from build123d import *

# Parameters (mm, degrees)
F1_DEPTH = 8
F2_R     = 2.5
F2_R_2   = 2
F3_DEPTH = 25
F5_DEPTH = 4
F7_DEPTH = 3
F8_R     = 0.5
F9_R     = 0.5


# Not quite as in the source:
# - a feature names something its author has since deleted; it is built from what else it names


with BuildPart() as f1:
    # F0 (on Top) → F1 (new body)
    with BuildSketch(Plane.XY):
        with BuildLine():
            Line((6.4761662253, 49.1160303571), (6.5, 49.6721517667))
            ThreePointArc((6.5, 49.6721517667), (0, 56.1721517667), (-6.5, 49.6721517667))
            Line((-6.5, 49.6721517667), (-6.4761662253, 49.1160303571))
            ThreePointArc((-6.4761662253, 49.1160303571), (0, 43.1721517667), (6.4761662253, 49.1160303571))
        make_face()
        with BuildLine():
            ThreePointArc((6.4761662253, 49.1160303571), (6.4940388228, 49.3938358172), (6.5, 49.6721517667))
            Line((6.5, 49.6721517667), (6.4761662253, 49.1160303571))
        make_face()
        with BuildLine():
            Line((-6.4761662253, 49.1160303571), (-6.5, 49.6721517667))
            ThreePointArc((-6.5, 49.6721517667), (-6.4940388228, 49.3938358172), (-6.4761662253, 49.1160303571))
        make_face()
        with BuildLine():
            Line((5, 14.6721517667), (6.4761662253, 49.1160303571))
            ThreePointArc((6.4761662253, 49.1160303571), (0, 43.1721517667), (-6.4761662253, 49.1160303571))
            Line((-6.4761662253, 49.1160303571), (-5, 14.6721517667))
            ThreePointArc((-5, 14.6721517667), (0, 19.6721517667), (5, 14.6721517667))
        make_face()
        with BuildLine():
            ThreePointArc((-5, 14.6721517667), (0, 9.6721517667), (5, 14.6721517667))
            ThreePointArc((5, 14.6721517667), (0, 19.6721517667), (-5, 14.6721517667))
        make_face()
    extrude(amount=F1_DEPTH)

    # F2 (on face) → F3 (cut)
    with BuildSketch(Plane.XY.offset(8)):
        with Locations((0, 49.6721517667)):
            Circle(F2_R)
        with Locations((0, 14.6721517667)):
            Circle(F2_R_2)
    extrude(amount=-F3_DEPTH, mode=Mode.SUBTRACT)

    # F4 (on face) → F5 (cut)
    with BuildSketch(Plane.XY.offset(8)):
        with BuildLine():
            Line((3.84, 48.5521517667), (4, 49.6721517667))
            ThreePointArc((4, 49.6721517667), (0, 53.6721517667), (-4, 49.6721517667))
            Line((-4, 49.6721517667), (-3.8313540205, 48.522923169))
            ThreePointArc((-3.8313540205, 48.522923169), (0.0152402747, 45.6721808001), (3.84, 48.5521517667))
        make_face()
        with BuildLine():
            ThreePointArc((3.84, 48.5521517667), (3.9597979746, 49.1064663418), (4, 49.6721517667))
            Line((4, 49.6721517667), (3.84, 48.5521517667))
        make_face()
        with BuildLine():
            Line((-3.8313540205, 48.522923169), (-4, 49.6721517667))
            ThreePointArc((-4, 49.6721517667), (-3.9576139328, 49.0913833455), (-3.8313540205, 48.522923169))
        make_face()
        with BuildLine():
            Line((2, 35.6721517667), (3.84, 48.5521517667))
            ThreePointArc((3.84, 48.5521517667), (0.0152402747, 45.6721808001), (-3.8313540205, 48.522923169))
            Line((-3.8313540205, 48.522923169), (-1.9833417846, 35.929747119))
            ThreePointArc((-1.9833417846, 35.929747119), (0.1290667091, 37.6679828679), (2, 35.6721517667))
        make_face()
        with BuildLine():
            ThreePointArc((-1.9833417846, 35.929747119), (-0.1290667091, 33.6763206655), (2, 35.6721517667))
            ThreePointArc((2, 35.6721517667), (0.1290667091, 37.6679828679), (-1.9833417846, 35.929747119))
        make_face()
    extrude(amount=-F5_DEPTH, mode=Mode.SUBTRACT)

    # F6 (on face) → F7 (cut)
    with BuildSketch(Plane.XY.offset(8)):
        with BuildLine():
            ThreePointArc((-4.1204651564, 17.5044241573), (0, 19.6721517667), (4.1204651564, 17.5044241573))
            Line((4.1204651564, 17.5044241573), (4.8918937278, 35.5044241573))
            ThreePointArc((4.8918937278, 35.5044241573), (0, 31.9420729635), (-4.8918937278, 35.5044241573))
            Line((-4.8918937278, 35.5044241573), (-4.1204651564, 17.5044241573))
        make_face()
    extrude(amount=-F7_DEPTH, mode=Mode.SUBTRACT)

    # F8
    f8_edges = [f1.edges().sort_by_distance(p)[0] for p in [
        (4.891894, 35.504424, 6.5),
    ]]
    fillet(f8_edges, radius=F8_R)

    # F9
    f9_edges = [f1.edges().sort_by_distance(p)[0] for p in [
        (-4.891894, 35.504424, 6.5),
        (4.120465, 17.504424, 6.5),
        (-4.120465, 17.504424, 6.5),
    ]]
    fillet(f9_edges, radius=F9_R)


solid = f1.part
Read the model definition and answer for the solid it produces. Units are mm, in the model's axes. A direction names the side the tool comes from. Round coordinates to 2 decimals unless told otherwise and drop trailing zeros. Order: outer loops, then holes, each group sorted by start corner. A loop starts at its lowest first (then second) coordinate and runs counter-clockwise, first axis right, second up. Notation, with made-up numbers: (-38.5, 33.25) - (9.5, 33.25) arc R22 ccw to (9.5, 53.25) - close; hole circle Ø6 at (21.25, 80). An arc over 180 degrees is marked (long way). Use one line per item in the form item = value. Start each with the question number.
(1) Determine the mould class of faces 3 (the face through (5.728, 31.653, 3.944)), 4 (the face through (0, 33, 0)), 5 (the face through (4.484, 25.976, 6.521)) for opening direction Y: +Y half, -Y half, draft (parallel to the pull), parting line (faces both ways), or undercut.
(2) Find the intervals of material crossed by line 1 along Y through (x, z) = (0, 2.6); line 2 along Y through (x, z) = (0, 4.5); line 3 along Z through (x, y) = (-0.5, 43), in increasing order. Write a range as from..to.
(3) The part is cut by section A-A (z = 5.5). Give the vertices of the cut face in (x, y).
(4) For faces 1 (the face through (1.344, 51.78, 2.028)), 2 (the face through (4.49, 33.9, 6.48)), determine the directions among +Z, -Z, +X, -X, +Y, -Y from which every point of the face is accessible in a straight line to the end or side of a thin tool.
(5) The part is cut by section C-C (z = 1.75). Give the vertices of the cut face in (x, y).
(6) The part is cut by section B-B (x = 0). Give the vertices of the cut face in (y, z).
(7) The part is cut by section D-D (y = 30). Give the vertices of the cut face in (x, z).
(8) Flat-ended cylindrical pins translate along their axes: pin 1 Ø2 at (y, z) = (41.5, 3.5) entering from +X; pin 2 Ø3 at (x, y) = (0, 49.67) entering from +Z; pin 3 Ø4 at (y, z) = (17, 5.5) entering from +X; pin 4 Ø2.5 at (x, y) = (1.5, 42) entering from +Z. Find the tip coordinate at first contact, or state that the pin passes through.
Checked values:
q1.face_3 = -Y half
q1.face_4 = draft
q1.face_5 = undercut
q2.line_1 = 9.67..12.67, 16.67..47.17, 52.17..56.17
q2.line_2 = 9.67..12.67, 16.67..33.67, 53.67..56.17
q2.line_3 = 0..4
q3.outline = (-6.48, 49.12) - (-5, 14.67) arc R5 ccw to (5, 14.67) - (6.48, 49.12) arc R6.5 ccw (long way) to start; hole (-4.8, 33.41) - (-4.17, 18.74) arc R0.5 ccw to (-3.34, 18.39) arc R5 cw to (3.34, 18.39) arc R0.5 ccw to (4.17, 18.74) - (4.8, 33.41) arc R0.5 ccw to (3.92, 33.76) arc R5.14 cw to (-3.92, 33.76) arc R0.5 ccw to start; hole (-3.83, 48.52) - (-1.98, 35.93) arc R2 ccw (long way) to (2, 35.67) - (3.84, 48.55) arc R4 ccw (long way) to start; hole circle Ø4 at (0, 14.67)
q4.face_1 = +Z, -Z
q4.face_2 = +Z
q5.outline = (-6.48, 49.12) - (-5, 14.67) arc R5 ccw to (5, 14.67) - (6.48, 49.12) arc R6.5 ccw (long way) to start; hole circle Ø5 at (0, 49.67); hole circle Ø4 at (0, 14.67)
q6.outline = (9.67, 0) - (12.67, 0) - (12.67, 8) - (9.67, 8) - close; (16.67, 0) - (47.17, 0) - (47.17, 4) - (33.67, 4) - (33.67, 8) - (31.94, 8) - (31.94, 5) - (19.67, 5) - (19.67, 8) - (16.67, 8) - close; (52.17, 0) - (56.17, 0) - (56.17, 8) - (53.67, 8) - (53.67, 4) - (52.17, 4) - close
q7.outline = (-5.66, 0) - (5.66, 0) - (5.66, 8) - (4.66, 8) - (4.66, 5) - (-4.66, 5) - (-4.66, 8) - (-5.66, 8) - close
q8.pin_1 = 6.19
q8.pin_2 = through
q8.pin_3 = 5.19
q8.pin_4 = 4
